For this review, take the finished solid that the model builds, in its own axes (mm). A direction names the side the tool comes from. Round coordinates to 2 decimals unless told otherwise and drop trailing zeros. Write each loop counter-clockwise with the first axis right and the second up, starting at its lowest first coordinate (ties: lowest second). Pieces come first, ordered by that corner, then holes.
from build123d import *

# Parameters (mm, degrees)
IZIM1_W                     = 150
IZIM1_H                     = 150
Y_KSEKLIK_EKSTR_ZYON1_DEPTH = 40
BO_ALTMA1_T                 = -4
IZIM2_W                     = 200
IZIM2_H                     = 200
IZIM2_W_2                   = 150
IZIM2_H_2                   = 150
Y_KSEKLIK_EKSTR_ZYON2_DEPTH = 4
KES_EKSTR_ZYON1_REACH       = 252.092
IZIM3_R                     = 5
KES_EKSTR_ZYON2_REACH       = 252.699
IZIM4_R                     = 2
IZIM4_W                     = 40
IZIM4_H                     = 20


with BuildPart() as part:
    # Çizim1 → Yükseklik-Ekstrüzyon1 (new body)
    with BuildSketch(Plane(origin=(0, 0, 0), x_dir=(1, 0, 0), z_dir=(0, 1, 0))):
        with Locations((-75, 75)):
            Rectangle(IZIM1_W, IZIM1_H)
    extrude(amount=Y_KSEKLIK_EKSTR_ZYON1_DEPTH)

    # İç Boşaltma1
    bo_altma1_openings = [part.faces().sort_by_distance(p)[0] for p in [
        (-75, 0, -75),
    ]]
    offset(amount=BO_ALTMA1_T, openings=bo_altma1_openings, kind=Kind.INTERSECTION)

    # Çizim2 → Yükseklik-Ekstrüzyon2 (add)
    with BuildSketch(Plane.XZ):
        with Locations((-75, -75)):
            Rectangle(IZIM2_W, IZIM2_H)
        with Locations((-75, -75)):
            Rectangle(IZIM2_W_2, IZIM2_H_2, mode=Mode.SUBTRACT)
    extrude(amount=-Y_KSEKLIK_EKSTR_ZYON2_DEPTH)

    # Çizim3 → Kes-Ekstrüzyon1 (cut, up to next)
    with BuildSketch(Plane(origin=(0, 4, 0), x_dir=(1, 0, 0), z_dir=(0, 1, 0)), mode=Mode.PRIVATE) as kes_ekstr_zyon1_sk1:
        with Locations(Location((12.5, 162.5, 0), (0, 0, 270))):
            Circle(IZIM3_R)
    kes_ekstr_zyon1_tool1 = extrude(kes_ekstr_zyon1_sk1.sketch, amount=-KES_EKSTR_ZYON1_REACH, mode=Mode.PRIVATE) & part.part
    # Çizim3 → Kes-Ekstrüzyon1 (cut, up to next)
    with BuildSketch(Plane(origin=(0, 4, 0), x_dir=(1, 0, 0), z_dir=(0, 1, 0)), mode=Mode.PRIVATE) as kes_ekstr_zyon1_sk2:
        with Locations(Location((12.5, -12.5, 0), (0, 0, 270))):
            Circle(IZIM3_R)
    kes_ekstr_zyon1_tool2 = extrude(kes_ekstr_zyon1_sk2.sketch, amount=-KES_EKSTR_ZYON1_REACH, mode=Mode.PRIVATE) & part.part
    # Çizim3 → Kes-Ekstrüzyon1 (cut, up to next)
    with BuildSketch(Plane(origin=(0, 4, 0), x_dir=(1, 0, 0), z_dir=(0, 1, 0)), mode=Mode.PRIVATE) as kes_ekstr_zyon1_sk3:
        with Locations(Location((-162.5, -12.5, 0), (0, 0, 270))):
            Circle(IZIM3_R)
    kes_ekstr_zyon1_tool3 = extrude(kes_ekstr_zyon1_sk3.sketch, amount=-KES_EKSTR_ZYON1_REACH, mode=Mode.PRIVATE) & part.part
    # Çizim3 → Kes-Ekstrüzyon1 (cut, up to next)
    with BuildSketch(Plane(origin=(0, 4, 0), x_dir=(1, 0, 0), z_dir=(0, 1, 0)), mode=Mode.PRIVATE) as kes_ekstr_zyon1_sk4:
        with Locations(Location((-162.5, 162.5, 0), (0, 0, 270))):
            Circle(IZIM3_R)
    kes_ekstr_zyon1_tool4 = extrude(kes_ekstr_zyon1_sk4.sketch, amount=-KES_EKSTR_ZYON1_REACH, mode=Mode.PRIVATE) & part.part
    add(kes_ekstr_zyon1_tool1.solids().sort_by_distance((12.5, 4, -162.5))[0], mode=Mode.SUBTRACT)
    add(kes_ekstr_zyon1_tool2.solids().sort_by_distance((12.5, 4, 12.5))[0], mode=Mode.SUBTRACT)
    add(kes_ekstr_zyon1_tool3.solids().sort_by_distance((-162.5, 4, 12.5))[0], mode=Mode.SUBTRACT)
    add(kes_ekstr_zyon1_tool4.solids().sort_by_distance((-162.5, 4, -162.5))[0], mode=Mode.SUBTRACT)

    # Çizim4 → Kes-Ekstrüzyon2 (cut, up to next)
    with BuildSketch(Plane(origin=(0, 40, 0), x_dir=(1, 0, 0), z_dir=(0, 1, 0)), mode=Mode.PRIVATE) as kes_ekstr_zyon2_sk1:
        with Locations(Location((-51.5, 70, 0), (0, 0, 270))):
            Circle(IZIM4_R)
    kes_ekstr_zyon2_tool1 = extrude(kes_ekstr_zyon2_sk1.sketch, amount=-KES_EKSTR_ZYON2_REACH, mode=Mode.PRIVATE) & part.part
    # Çizim4 → Kes-Ekstrüzyon2 (cut, up to next)
    with BuildSketch(Plane(origin=(0, 40, 0), x_dir=(1, 0, 0), z_dir=(0, 1, 0)), mode=Mode.PRIVATE) as kes_ekstr_zyon2_sk2:
        with Locations(Location((-51.5, 80, 0), (0, 0, 270))):
            Circle(IZIM4_R)
    kes_ekstr_zyon2_tool2 = extrude(kes_ekstr_zyon2_sk2.sketch, amount=-KES_EKSTR_ZYON2_REACH, mode=Mode.PRIVATE) & part.part
    # Çizim4 → Kes-Ekstrüzyon2 (cut, up to next)
    with BuildSketch(Plane(origin=(0, 40, 0), x_dir=(1, 0, 0), z_dir=(0, 1, 0)), mode=Mode.PRIVATE) as kes_ekstr_zyon2_sk3:
        with Locations(Location((-98.5, 80, 0), (0, 0, 270))):
            Circle(IZIM4_R)
    kes_ekstr_zyon2_tool3 = extrude(kes_ekstr_zyon2_sk3.sketch, amount=-KES_EKSTR_ZYON2_REACH, mode=Mode.PRIVATE) & part.part
    # Çizim4 → Kes-Ekstrüzyon2 (cut, up to next)
    with BuildSketch(Plane(origin=(0, 40, 0), x_dir=(1, 0, 0), z_dir=(0, 1, 0)), mode=Mode.PRIVATE) as kes_ekstr_zyon2_sk4:
        with Locations(Location((-98.5, 70, 0), (0, 0, 270))):
            Circle(IZIM4_R)
    kes_ekstr_zyon2_tool4 = extrude(kes_ekstr_zyon2_sk4.sketch, amount=-KES_EKSTR_ZYON2_REACH, mode=Mode.PRIVATE) & part.part
    # Çizim4 → Kes-Ekstrüzyon2 (cut, up to next)
    with BuildSketch(Plane(origin=(0, 40, 0), x_dir=(1, 0, 0), z_dir=(0, 1, 0)), mode=Mode.PRIVATE) as kes_ekstr_zyon2_sk5:
        with Locations((-75, 75)):
            Rectangle(IZIM4_W, IZIM4_H)
    kes_ekstr_zyon2_tool5 = extrude(kes_ekstr_zyon2_sk5.sketch, amount=-KES_EKSTR_ZYON2_REACH, mode=Mode.PRIVATE) & part.part
    add(kes_ekstr_zyon2_tool1.solids().sort_by_distance((-51.5, 40, -70))[0], mode=Mode.SUBTRACT)
    add(kes_ekstr_zyon2_tool2.solids().sort_by_distance((-51.5, 40, -80))[0], mode=Mode.SUBTRACT)
    add(kes_ekstr_zyon2_tool3.solids().sort_by_distance((-98.5, 40, -80))[0], mode=Mode.SUBTRACT)
    add(kes_ekstr_zyon2_tool4.solids().sort_by_distance((-98.5, 40, -70))[0], mode=Mode.SUBTRACT)
    add(kes_ekstr_zyon2_tool5.solids().sort_by_distance((-75, 40, -75))[0], mode=Mode.SUBTRACT)


solid = part.part
(1) We need section A-A, the plane y = 24. Give the boundary of the cut face in (x, z).
Geometry check:
outline: (-150, -150) - (0, -150) - (0, 0) - (-150, 0) - close; hole (-146, -146) - (-4, -146) - (-4, -4) - (-146, -4) - close
(2) For faces 1 (the face through (0, 22, -74)), 2 (the face through (-76, 22, -150)), 3 (the face through (-76, 18, -4)), list the 3-axis set-ups (+Z, -Z, +X, -X, +Y, -Y) from which the entire face can be reached by the end or side of a thin tool; tool diameter is ignored.
Geometry check:
face 1: +Z, -Z, +X, +Y
face 2: -Z, +X, -X, +Y
face 3: -Y
(3) We need section D-D, the plane x = 12.5. Give the boundary of the cut face in (y, z), and give its area (3 significant figures).
Geometry check:
outline: (0, -175) - (4, -175) - (4, -167.5) - (0, -167.5) - close; (0, -157.5) - (4, -157.5) - (4, 7.5) - (0, 7.5) - close; (0, 17.5) - (4, 17.5) - (4, 25) - (0, 25) - close
area: 720 mm2
(4) For line 1 along X through (y, z) = (37.85, -80); line 2 along X through (y, z) = (16.5, -103), list the stretches that pass through material, from the lowest coordinate up.
Geometry check:
line 1: x = -150 to -100.5, -96.5 to -95, -55 to -53.5, -49.5 to 0
line 2: x = -150 to -146, -4 to 0
(5) We need section B-B, the plane x = -90.5. Give the boundary of the cut face in (y, z), and give its area (3 significant figures).
Geometry check:
outline: (0, -175) - (4, -175) - (4, -150) - (40, -150) - (40, -85) - (36, -85) - (36, -146) - (0, -146) - close; (0, -4) - (36, -4) - (36, -65) - (40, -65) - (40, 0) - (4, 0) - (4, 25) - (0, 25) - close
area: 1,010 mm2
(6) For pin 1 Ø4.5 at (x, y) = (-72, 38) entering from +Z; pin 2 Ø1.5 at (y, z) = (18, -13.5) entering from +X; pin 3 Ø11 at (y, z) = (27, -106.5) entering from -X, all flat-tipped, find the tip position at first contact; note any pin that passes through.
Geometry check:
pin 1: stops at z = 0
pin 2: stops at x = 0
pin 3: stops at x = -150
(7) We need section C-C, the plane z = -162.5. Give the boundary of the cut face in (x, y).
Geometry check:
outline: (-175, 0) - (-167.5, 0) - (-167.5, 4) - (-175, 4) - close; (-157.5, 0) - (7.5, 0) - (7.5, 4) - (-157.5, 4) - close; (17.5, 0) - (25, 0) - (25, 4) - (17.5, 4) - close
(8) Mouldability with a two-part tool opening along X and no side actions: class faces 4 (the face through (-76, 36, -60)), 5 (the face through (-76, 22, 0)), 6 (the face through (-150, 22, -74)) as pulls with the +X half, pulls with the -X half, needs draft (parallel to the pull), parting line crosses it, or undercut.
Geometry check:
face 4: undercut
face 5: needs draft
face 6: pulls with the -X half
